from build123d import *

# Parameters (mm, degrees)
SKETCH1_R          = 6.8834
EXTRUDE1_DEPTH     = 10.668
SKETCH1_2_R        = 6.8834
EXTRUDE2_DEPTH     = 2.032
SKETCH3_R          = 1.905
CUT_EXTRUDE1_DEPTH = 6.35
EXTRUDE3_DEPTH     = 5.842
SKETCH5_R          = 7.9375
EXTRUDE4_DEPTH     = 46.736
SKETCH6_R          = 6.1515625
EXTRUDE5_DEPTH     = 8.334375
SKETCH7_R          = 4.1671875
EXTRUDE6_DEPTH     = 12.7


with BuildPart() as part:
    # Sketch1 → Extrude1 (new body)
    with BuildSketch(Plane.XY):
        Circle(SKETCH1_R)
    extrude(amount=EXTRUDE1_DEPTH)

    # Sketch2 → Cut-Revolve5 (revolve, cut)
    with BuildSketch(Plane(origin=(0, 0, 0), x_dir=(0, 0, -1), z_dir=(1, 0, 0))):
        Polygon((-10.668, 6.8834), (-9.672936951, 5.888336951), (-8.802379845, 6.758894057), (-7.921944961, 5.878459173), (-7.041510078, 6.758894057), (-6.089928941, 5.80731292), (-5.138347804, 6.758894057), (-4.15119354, 5.771739793), (-3.164039276, 6.758894057), (-2.248031266, 5.842886047), (-1.332023256, 6.758894057), (-0.514702762, 5.941573563), (0, 6.8834), align=None)
    revolve(axis=Axis((0, 0, 12.00396124), (0, 0, -1)), mode=Mode.SUBTRACT)

    # Sketch1<2> → Extrude2 (add)
    with BuildSketch(Plane.XY):
        Circle(SKETCH1_2_R)
    extrude(amount=-EXTRUDE2_DEPTH)

    # Sketch3 → Cut-Extrude1 (cut)
    with BuildSketch(Plane.XY.offset(10.668)):
        Circle(SKETCH3_R)
    extrude(amount=-CUT_EXTRUDE1_DEPTH, mode=Mode.SUBTRACT)

    # Sketch4 → Extrude3 (add)
    with BuildSketch(Plane(origin=(0, 0, -2.032), x_dir=(-1, 0, 0), z_dir=(0, 0, -1))):
        Polygon((-4.582717762, 7.9375), (4.582717762, 7.9375), (9.165435523, 0), (4.582717762, -7.9375), (-4.582717762, -7.9375), (-9.165435523, 0), align=None)
    extrude(amount=EXTRUDE3_DEPTH)

    # Sketch5 → Extrude4 (add)
    with BuildSketch(Plane(origin=(0, 0, -7.874), x_dir=(-1, 0, 0), z_dir=(0, 0, -1))):
        Circle(SKETCH5_R)
    extrude(amount=EXTRUDE4_DEPTH)

    # Sketch6 → Extrude5 (add)
    with BuildSketch(Plane(origin=(0, 0, -54.61), x_dir=(-1, 0, 0), z_dir=(0, 0, -1))):
        Circle(SKETCH6_R)
    extrude(amount=EXTRUDE5_DEPTH)

    # Sketch7 → Extrude6 (add)
    with BuildSketch(Plane(origin=(0, 0, -62.944375), x_dir=(-1, 0, 0), z_dir=(0, 0, -1))):
        Circle(SKETCH7_R)
    extrude(amount=EXTRUDE6_DEPTH)


solid = part.part
Here's how the part is built. I have some questions about the finished solid (model axes, mm). A direction names the side the tool comes from. Coordinates: 2 decimals unless noted, no trailing zeros. Order: outer loops, then holes, each group sorted by start corner. A loop starts at its lowest first (then second) coordinate and runs counter-clockwise, first axis right, second up. Notation, with made-up numbers: M -7,72 L 16,72 A12 cw 16,85 Z; hole C -1.75,-16.75 d7. An arc over 180 degrees is marked long. Answer as CSV lines item,"result". Start each with the question number.
1. On a 3-axis mill with a long thin cutter (end or side, diameter ignored), from which of +Z, -Z, +X, -X, +Y, -Y can I reach the whole of each face in a straight line? I mean faces 1 (the flat face through (-4, -5, -54.61)), 2 (the flat face through (7, 2, -2.032)), 3 (the flat face through (8.3, 0, -7.874)), 4 (the flat face through (-4, 7.1, -7.874)). Say none if no direction works.
2. I need wall thicknesses on line 1 (Z direction, x = -6.25, y = 3); line 2 (Y direction, x = 0, z = 7.75) (3 decimals); line 3 (Y direction, x = 0, z = 8) (3 decimals). Which ranges of each line are inside material? Lowest first, please. Write a range as [from, to].
3. I want a section at A-A, the plane z = -19.5. Write out the boundary of the cut face in (x, y) (1 decimal).
4. For pin 1 (2 mm diameter, centred on x = 2, y = 6.5, fed in from -Z); pin 2 (1.2 mm diameter, centred on x = -4, y = -5.5, fed in from -Z); pin 3 (2 mm diameter, centred on y = 5, z = -22.5, fed in from +X), each with a flat end and sliding along its axis, tell me the tip position at first contact or that it passes through.
Recorded:
1,face 1,"-Z"
1,face 2,"+Z"
1,face 3,"-Z, +X"
1,face 4,"-Z, -X, +Y"
2,line 1,"z = [-54.61, -2.03]"
2,line 2,"y = [-6.05, -1.905], [1.905, 6.05]"
2,line 3,"y = [-5.957, -1.905], [1.905, 5.957]"
3,outline,"C 0,0 d15.9"
4,pin 1,"stops at z = -62.94"
4,pin 2,"stops at z = -54.61"
4,pin 3,"stops at x = 6.86"
